```python
from build123d import *

# Parameters (mm, degrees)
F1_DEPTH = 2.5
F2_W     = 41.65861
F2_H     = 13.999665
F3_DEPTH = 25


with BuildPart() as f1:
    # F0 (on Front) → F1 (new body, symmetric)
    with BuildSketch(Plane.XZ):
        Polygon((-34.5, 0), (-34.5, -59), (33.5, -59), (33.5, 35), (0, 35), align=None)
    extrude(amount=F1_DEPTH, both=True)

    # F2 (on face) → F3 (cut)
    with BuildSketch(Plane.XZ.offset(2.5)):
        with Locations((-0.598928, -6.999833)):
            Rectangle(F2_W, F2_H)
    extrude(amount=-F3_DEPTH, mode=Mode.SUBTRACT)


solid = f1.part
```
Input: part model. Units: mm. Frame: model coordinates. A direction names the side the tool comes from. Coordinates: 2 decimals unless noted, no trailing zeros. Write each loop counter-clockwise with the first axis right and the second up, starting at its lowest first coordinate (ties: lowest second). Pieces come first, ordered by that corner, then holes. Notation, with made-up numbers: M -31,-15 L 7,-15 A25 cw 7,24 Z; hole C -19.5,-25.5 d4. An arc over 180 degrees is marked long. Use one line per item in the form item = value.
Q1. Set-up query: faces 1 (the face through (-1, 0, -14)), 2 (the face through (-1, -2.5, -22)). Return all of +Z, -Z, +X, -X, +Y, -Y with unobstructed straight access to the full face (end or side cutting, diameter ignored); none if empty.
Answer below:
face_1 = +Y, -Y
face_2 = +Z, -Z, +X, -X, -Y
Q2. Material intervals for probe 1 along Z at (x, y) = (7.5, 1.4); probe 2 along X at (y, z) = (-1.35, -11.5); probe 3 along Z at (x, y) = (-7, 2.25), sorted ascending. Write a range as from..to.
Answer below:
probe_1 = -59..-14, 0..35
probe_2 = -34.5..-21.43, 20.23..33.5
probe_3 = -59..-14, 0..27.9
Q3. First-contact query: pin 1 (1.5 mm diameter, centred on y = -1, z = 24, fed in from -X). Flat tip, straight axial feed; report the tip coordinate or a pass-through.
Answer below:
pin_1 = -11.58
Q4. Section A-A (y = 0.3). Return loops of the section in (x, z), plus the area to 3 significant figures.
Answer below:
outline = M -34.5,-59 L 33.5,-59 L 33.5,35 L 0,35 L -34.5,0 Z; hole M -21.43,-14 L 20.23,-14 L 20.23,0 L -21.43,0 Z
area = 5,210 mm²
Q5. Section C-C (z = -8). Return loops of the section in (x, y), plus the area to 3 significant figures.
Answer below:
outline = M -34.5,-2.5 L -21.43,-2.5 L -21.43,2.5 L -34.5,2.5 Z; M 20.23,-2.5 L 33.5,-2.5 L 33.5,2.5 L 20.23,2.5 Z
area = 132 mm²
Q6. Section D-D (z = 16). Return loops of the section in (x, y).
Answer below:
outline = M -18.73,-2.5 L 33.5,-2.5 L 33.5,2.5 L -18.73,2.5 Z
Q7. Draft query along X for faces 3 (the face through (-1, 0, 0)), 4 (the face through (-1, 0, -59)), 5 (the face through (-34.5, 0, -29)). Return one class per face: released by +X, released by -X, zero draft, split by the parting line, or undercut.
Answer below:
face_3 = undercut
face_4 = zero draft
face_5 = released by -X
Q8. Section B-B (x = 14). Return loops of the section in (y, z), plus the area to 3 significant figures.
Answer below:
outline = M -2.5,-59 L 2.5,-59 L 2.5,-14 L -2.5,-14 Z; M -2.5,0 L 2.5,0 L 2.5,35 L -2.5,35 Z
area = 400 mm²
